Print and shaded views of the part. All mm, measured from the part's lowest x, y and z. Round coordinates to 2 decimals unless told otherwise and drop trailing zeros. Order: outer loops, then holes, each group sorted by start corner. A loop starts at its lowest first (then second) coordinate and runs counter-clockwise, first axis right, second up. Notation, with made-up numbers: M 52.25,-14.75 L 78.25,-14.75 A19 ccw 78.25,5.25 Z; hole C -30,-17.5 d10. An arc over 180 degrees is marked long. Use CSV: the item, a comma, the result in double quotes.
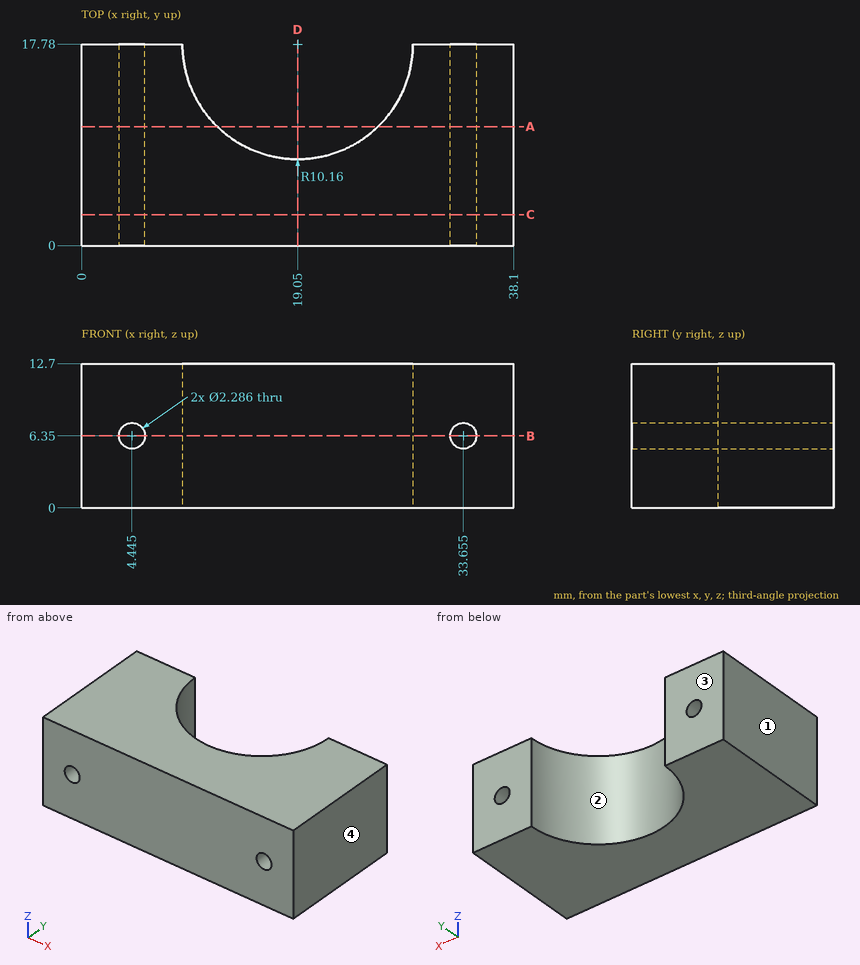
(1) Cut at A-A, the plane y = 10.5. Give the cut face in (x, z) (3 decimals), and give its area (3 significant figures).
Answer block:
outline,"M 0,0 L 11.963,0 L 11.963,12.7 L 0,12.7 Z; M 26.137,0 L 38.1,0 L 38.1,12.7 L 26.137,12.7 Z; hole C 4.445,6.35 d2.286; hole C 33.655,6.35 d2.286"
area,"296 mm²"
(2) Wall check: line 1 (X direction, y = 12, z = 11); line 2 (X direction, y = 12.75, z = 1.75); line 3 (Z direction, x = 34, y = 4.75). Give the ranges that are in metal, low to high. Write a range as from..to.
Answer block:
line 1,"x = 0..10.69, 27.41..38.1"
line 2,"x = 0..10.22, 27.88..38.1"
line 3,"z = 0..5.26, 7.44..12.7"
(3) Drop a flat-ended pin along its axis: pin 1 (6 mm diameter, centred on x = 28, y = 9.5, fed in from -Z). Give the stop position or say it passes through.
Answer block:
pin 1,"stops at z = 0"
(4) Cut at D-D, the plane x = 19.05. Give the cut face in (y, z).
Answer block:
outline,"M 0,0 L 7.62,0 L 7.62,12.7 L 0,12.7 Z"
(5) Cut at C-C, the plane y = 2.75. Give the cut face in (x, z) (3 decimals).
Answer block:
outline,"M 0,0 L 38.1,0 L 38.1,12.7 L 0,12.7 Z; hole C 4.445,6.35 d2.286; hole C 33.655,6.35 d2.286"
(6) Two-plate mould, pull along X, no slides. Class the marked faces 1, 2, 3 and 4: released by +X, released by -X, zero draft, split by the parting line, or undercut.
Answer block:
face 1,"released by -X"
face 2,"undercut"
face 3,"zero draft"
face 4,"released by +X"
(7) Cut at B-B, the plane z = 6.35. Give the cut face in (x, y), and give its area (3 significant figures).
Answer block:
outline,"M 0,0 L 3.3,0 L 3.3,17.78 L 0,17.78 Z; M 5.59,0 L 32.51,0 L 32.51,17.78 L 29.21,17.78 A10.16 cw 8.89,17.78 L 5.59,17.78 Z; M 34.8,0 L 38.1,0 L 38.1,17.78 L 34.8,17.78 Z"
area,"434 mm²"
